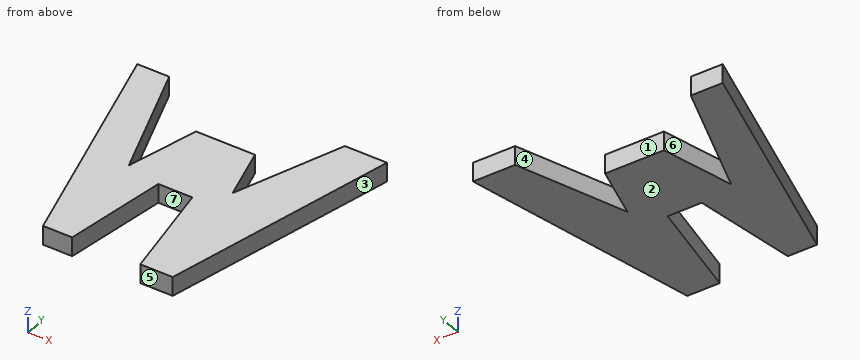
```python
from build123d import *

# Parameters (mm, degrees)
F0_W     = 84.4042
F0_H     = 79.8273328692
F1_DEPTH = 6.35
F3_DEPTH = 25.4


with BuildPart() as f1:
    # F0 (on Top) → F1 (new body)
    with BuildSketch(Plane.XY):
        with Locations((1.090981224, 11.9649684057)):
            Rectangle(F0_W, F0_H)
    extrude(amount=F1_DEPTH)

    # F2 (on face) → F3 (cut)
    with BuildSketch(Plane.XY.offset(6.35)):
        Polygon((-17.5364390016, -27.9486980289), (-41.111118776, 51.8786348402), (-41.111118776, -27.9486980289), align=None)
        Polygon((29.0447268635, 51.8786348403), (-30.3234253079, 51.8786348403), (-14.7963697091, 9.864247404), (-8.9508909732, 34.1595225036), (10.960274376, 34.1595225036), (16.5489539437, 15.2354315543), align=None)
        Polygon((43.293081224, -27.9486980289), (43.293081224, 51.8786348403), (26.3046585023, -27.9486980289), align=None)
        Polygon((-2.9227398336, 7.1241795085), (-7.6721920632, -27.9486980289), (15.3443841264, -27.9486980289), (8.5855480283, 7.1241795085), align=None)
    extrude(amount=-F3_DEPTH, mode=Mode.SUBTRACT)


solid = f1.part
```
Geometry: final body of the model. Coordinates: model frame, mm. Face numbers are marked on the shaded views. A direction names the side the tool comes from. Give positions to 0.01 mm unless a question says otherwise; leave off trailing zeros. Write each loop counter-clockwise with the first axis right and the second up, starting at its lowest first coordinate (ties: lowest second). Pieces come first, ordered by that corner, then holes.
1. Section query B-B, the plane z = 2.75. Return loops of the section in (x, y).
2. Reachability of the marked faces 5, 6 and 7 from +Z, -Z, +X, -X, +Y, -Y: full face, straight path, thin tool, end or side. Return the list, or none.
3. Draft query along X for the marked faces 1, 2, 3 and 4. Return one class per face: released by +X, released by -X, zero draft, split by the parting line, or undercut.
4. Pin query (flat end, axial travel): P1, Ø4, axis at x = 25.5, y = 30.5, coming from the -Z side; P2, Ø1, axis at y = 0.5, z = 2, coming from the -X side. Return the tip coordinate at first contact, or that it passes through.
5. Line query: probe 1 along Y at (x, z) = (-2, 3.75); probe 2 along X at (y, z) = (48, 6.25); probe 3 along X at (y, z) = (-24, 2.5) (3 decimals). Output: solid intervals per line, ascending.
6. Section query A-A, the plane y = 27. Return loops of the section in (x, z).
7. Section query C-C, the plane y = -7.5. Return loops of the section in (x, z), then the cut area to 3 significant figures.
8. Section query D-D, the plane x = 4.5. Return loops of the section in (y, z), then the cut area to 3 significant figures.
Computed:
1. outline: (-41.11, 51.88) - (-17.54, -27.95) - (-7.67, -27.95) - (-2.92, 7.12) - (8.59, 7.12) - (15.34, -27.95) - (26.3, -27.95) - (43.29, 51.88) - (29.04, 51.88) - (16.55, 15.24) - (10.96, 34.16) - (-8.95, 34.16) - (-14.8, 9.86) - (-30.32, 51.88) - close
2. face 5: +Z, -Z, +X, -X, -Y
2. face 6: +Z, -Z, +Y
2. face 7: +Z, -Z, -Y
3. face 1: undercut
3. face 2: zero draft
3. face 3: released by +X
3. face 4: undercut
4. P1: stops at z = 0
4. P2: stops at x = -26.09
5. probe 1: y = 7.12 to 34.16
5. probe 2: x = -39.97 to -28.89, 27.72 to 42.47
5. probe 3: x = -18.703 to -7.137, 14.583 to 27.145
6. outline: (-33.76, 0) - (-21.13, 0) - (-21.13, 6.35) - (-33.76, 6.35) - close; (-10.67, 0) - (13.07, 0) - (13.07, 6.35) - (-10.67, 6.35) - close; (20.56, 0) - (38, 0) - (38, 6.35) - (20.56, 6.35) - close
7. outline: (-23.58, 0) - (-4.9, 0) - (-4.9, 6.35) - (-23.58, 6.35) - close; (11.4, 0) - (30.66, 0) - (30.66, 6.35) - (11.4, 6.35) - close
7. area: 241 mm2
8. outline: (7.12, 0) - (34.16, 0) - (34.16, 6.35) - (7.12, 6.35) - close
8. area: 172 mm2
